from build123d import *

# Parameters (mm, degrees)
SKETCH1_W           = 28
SKETCH1_H           = 22
BOSS_EXTRUDE1_DEPTH = 1.5
SKETCH2_W           = 3.9
SKETCH2_H           = 4.9
BOSS_EXTRUDE2_DEPTH = 1.75
SKETCH3_R           = 1.3
CUT_EXTRUDE1_DEPTH  = 1.75


with BuildPart() as part:
    # Sketch1 → Boss-Extrude1 (new body)
    with BuildSketch(Plane(origin=(0, 0, 0), x_dir=(1, 0, 0), z_dir=(0, 1, 0))):
        Rectangle(SKETCH1_W, SKETCH1_H)
    extrude(amount=BOSS_EXTRUDE1_DEPTH)

    # Sketch2 → Boss-Extrude2 (add)
    with BuildSketch(Plane(origin=(0, 1.5, 0), x_dir=(1, 0, 0), z_dir=(0, 1, 0))):
        with Locations((6.5, 0)):
            Rectangle(SKETCH2_W, SKETCH2_H)
    extrude(amount=BOSS_EXTRUDE2_DEPTH)

    # Sketch3 → Cut-Extrude1 (cut)
    with BuildSketch(Plane(origin=(0, 1.5, 0), x_dir=(1, 0, 0), z_dir=(0, 1, 0))):
        with Locations(Location((12, -9, 0), (0, 0, 270))):
            Circle(SKETCH3_R)
        with Locations(Location((1, -9, 0), (0, 0, 270))):
            Circle(SKETCH3_R)
        with Locations(Location((12, 9, 0), (0, 0, 90))):
            Circle(SKETCH3_R)
        with Locations(Location((1, 9, 0), (0, 0, 90))):
            Circle(SKETCH3_R)
    extrude(amount=-CUT_EXTRUDE1_DEPTH, mode=Mode.SUBTRACT)


solid = part.part
The listing builds one solid part. Answer for the finished solid, in the listing's coordinates (mm). A direction names the side the tool comes from. Coordinates: 2 decimals unless noted, no trailing zeros. Order: outer loops, then holes, each group sorted by start corner. A loop starts at its lowest first (then second) coordinate and runs counter-clockwise, first axis right, second up.
Q1. A cutting plane is placed at B-B, the plane x = 12. Write down the section's boundary in (y, z).
Q2. Given P1, Ø5, axis at x = 1.5, z = 3, coming from the +Y side; P2, Ø1.5, axis at x = 2.5, z = 8, coming from the -Y side; P3, Ø1.9, axis at y = 2.5, z = 0.5, coming from the +X side; P4, Ø0.9, axis at x = 6.5, y = 2.5, coming from the -Z side, each flat-ended and moving along its own axis, determine where each tip first touches the part or whether it passes through.
Q3. A cutting plane is placed at C-C, the plane y = 1.15. Write down the section's boundary in (x, z).
Q4. A cutting plane is placed at A-A, the plane z = -8.5. Write down the section's boundary in (x, y), and give its area (3 significant figures).
Q5. For a pull along Z with two mould halves and no side action, classify faces 6 (the face through (0.61, 0.76, -10.24)), 7 (the face through (4.55, 2, 0)), 8 (the face through (0, 1, -11)) as pulls with the +Z half, pulls with the -Z half, needs draft (parallel to the pull), parting line crosses it, or undercut.
Q6. Which of the six approach directions +Z, -Z, +X, -X, +Y, -Y give full straight-line access (tool end or side, diameter ignored) to faces 1 (the face through (13.096, 0.76, 9.699)), 2 (the face through (6, 2, 2.45)), 3 (the face through (8.45, 2, 0)), 4 (the face through (6, 2, -2.45)), 5 (the face through (6, 3.25, 0))?
Q7. Consider line 1 (X direction, y = 0.45, z = -9); line 2 (Y direction, x = 4, z = -5.25); line 3 (X direction, y = 2.7, z = 0). Determine where each line is inside the solid, lowest interval first.
Q8. A cutting plane is placed at D-D, the plane z = -1.5. Write down the section's boundary in (x, y), and give its area (3 significant figures).
Answers follow:
1. outline: (0, -11) - (1.5, -11) - (1.5, -10.3) - (0, -10.3) - close; (0, -7.7) - (1.5, -7.7) - (1.5, 7.7) - (0, 7.7) - close; (0, 10.3) - (1.5, 10.3) - (1.5, 11) - (0, 11) - close
2. P1: stops at y = 1.5
2. P2: stops at y = 0
2. P3: stops at x = 8.45
2. P4: stops at z = -2.45
3. outline: (-14, -11) - (14, -11) - (14, 11) - (-14, 11) - close; hole circle Ø2.6 at (1, -9); hole circle Ø2.6 at (1, 9); hole circle Ø2.6 at (12, -9); hole circle Ø2.6 at (12, 9)
4. outline: (-14, 0) - (-0.2, 0) - (-0.2, 1.5) - (-14, 1.5) - close; (2.2, 0) - (10.8, 0) - (10.8, 1.5) - (2.2, 1.5) - close; (13.2, 0) - (14, 0) - (14, 1.5) - (13.2, 1.5) - close
4. area: 34.8 mm2
5. face 6: undercut
5. face 7: needs draft
5. face 8: pulls with the -Z half
6. face 1: +Y, -Y
6. face 2: +Z, +X, -X, +Y
6. face 3: +Z, -Z, +X, +Y
6. face 4: -Z, +X, -X, +Y
6. face 5: +Z, -Z, +X, -X, +Y
7. line 1: x = -14 to -0.3, 2.3 to 10.7, 13.3 to 14
7. line 2: y = 0 to 1.5
7. line 3: x = 4.55 to 8.45
8. outline: (-14, 0) - (14, 0) - (14, 1.5) - (8.45, 1.5) - (8.45, 3.25) - (4.55, 3.25) - (4.55, 1.5) - (-14, 1.5) - close
8. area: 48.8 mm2
